Autodesk Inventor part; units mm, degrees
ref_plane "Work Plane1" through (0, 0, 0) normal (0, 0, 1) x (1, 0, 0)
ref_plane "Work Plane2" through (0, 0, 122.75) normal (0, 0, 1) x (1, 0, 0)
ref_plane "YZ Plane" through (0, 0, 0) normal (1, 0, 0) x (0, 1, 0)
ref_plane "Work Plane1" through (0, 0, 0) normal (0, 0, 1) x (1, 0, 0)
sketch "Sketch1" plane through (0, 0, 0) normal (0, 0, 1) x (1, 0, 0)
  line L0 (10, 0) -> (-1.5, 0)
  line L1 (10, 45.2667) -> (10, 0)
  arc A0 (13.0769, 49.8821) -> (10, 45.2667) centre (15, 45.2667) ccw
  line L2 (54.8615, 67.2923) -> (13.0769, 49.8821)
  line L3 (50.4385, 77.9077) -> (54.8615, 67.2923)
  line L4 (50.4385, 77.9077) -> (29.2692, 69.0872)
  arc A1 (29.2692, 69.0872) -> (-1.5, 22.9333) centre (48.5, 22.9333) ccw
  line L5 (-1.5, 0) -> (-1.5, 22.9333)
  line L6 (15, 45.2667) -> (6.8975, 50.6683)
  line L7 (10, 48.6) -> (19.7692, 25.1538)
  line L8 (35.4, 31.6667) -> (10, 21.0833)
  line L9 (19.1124, 26.7302) -> (10, 22.9333)
  line L10 (-1.5, 22.9333) -> (10, 22.9333)
  line L11 (-1.5, 22.9333) -> (0, 22.9333)
  line L12 (0, 22.9333) -> (0, -23.4445)
  line L13 (0, -23.4445) -> (-1.5, -23.4445)
  line L14 (-1.5, -23.4445) -> (-1.5, 22.9333)
  line L15 (0, 0.0333) -> (4, 0.0333)
  line L16 (4, 0.0333) -> (10, 6.0333)
  point P0 (0, 0)
  point P1 (10.4897, 47.4247)
  point P2 (10.8397, 48.0402)
  point P3 (10, 48.6)
  point P4 (0, 22.9333)
  dimension "d3" = 1.5
  dimension "d4" = 4
  dimension "d5" = 45
  dimension "d6" = 22.9
extrude "Extrusion1" add sketch "Sketch1" along normal blind 245.5 contours L16 L15 L12 L10 L1 | A1 L6 L7 A0 L1 L10 | L1 A0 L7 L9 | L6 A0 L7
sketch "Sketch2" plane through (6.8975, 50.6683, 245.5) normal (0.5547, 0.8321, 0) x (0.8321, -0.5547, 0)
  line L0 (4.738, 245.5) -> (0, 245.5)
  line L1 (0, 245.5) -> (0, 0)
  line L2 (4.738, 0) -> (0, 0)
  line L3 (4.738, 245.5) -> (4.738, 0)
  circle A0 centre (2.5, 230.5) radius 1.25
  circle A1 centre (2.5, 180.5) radius 1.25
  circle A2 centre (2.5, 130.5) radius 1.25
  circle A3 centre (2.5, 80.5) radius 1.25
  circle A4 centre (2.5, 30.5) radius 1.25
  point P0 (22.3667, 245.5)
  dimension "d7" = 2.5
  dimension "d8" = 2.5
  dimension "d9" = 15
  dimension "d12" = 50
extrude "Extrusion2" cut sketch "Sketch2" against normal blind 3 contours A0 | A1 | A2 | A3 | A4
sketch "Sketch3" plane through (0, 0, 0) normal (0, 0, -1) x (-1, 0, 0)
  line L0 (-10, 6.0333) -> (-10, 22.9333)
  line L1 (-4, 0.0333) -> (-10, 6.0333)
  line L2 (0, 0.0333) -> (-4, 0.0333)
  line L3 (0, 22.9333) -> (0, 0.0333)
  line L4 (1.5, 22.9333) -> (0, 22.9333)
  arc A0 (1.5, 22.9333) -> (-6.8975, 50.6683) centre (-48.5, 22.9333) ccw
  line L5 (-10.8397, 48.0402) -> (-6.8975, 50.6683)
  arc A1 (-10.4897, 47.4247) -> (-10.8397, 48.0402) centre (-15, 45.2667) ccw
  line L6 (-19.1124, 26.7302) -> (-10.4897, 47.4247)
  line L7 (-10, 22.9333) -> (-19.1124, 26.7302)
  line L8 (-12.4384, 34.9479) -> (-14.7461, 29.4095)
  line L9 (-14.7461, 29.4095) -> (-11.9768, 28.2556)
  line L10 (-11.9768, 28.2556) -> (-9.6691, 33.7941)
  line L11 (-9.6691, 33.7941) -> (-12.4384, 34.9479)
  point P0 (0, 0)
  dimension "d19" = 12.7
  dimension "d20" = 6
  dimension "d21" = 3
  dimension "d22" = 3
extrude "Extrusion3" cut sketch "Sketch3" against normal blind 30 contours L11 L10 L9 L8
sketch "Sketch4" plane through (10.4897, 47.4247, 245.5) normal (0.9231, 0.3846, 0) x (0, 0, -1)
  line L0 (245.5, -22.4191) -> (245.5, 0)
  line L1 (245.5, 0) -> (0, 0)
  line L2 (0, -22.4191) -> (0, 0)
  line L3 (245.5, -22.4191) -> (0, -22.4191)
  line L4 (245.5, -18.2665) -> (245.5, -12.2665) construction
  line L5 (245.5, -18.2665) -> (215.5, -18.2665)
  line L6 (215.5, -18.2665) -> (215.5, -12.2665)
  line L7 (245.5, -12.2665) -> (215.5, -12.2665)
  circle A0 centre (219.1, -15.2665) radius 1.65
  line L8 (220.7743, -18.1665) -> (217.4257, -18.1665)
  line L9 (217.4257, -18.1665) -> (215.7514, -15.2665)
  line L10 (215.7514, -15.2665) -> (217.4257, -12.3665)
  line L11 (217.4257, -12.3665) -> (220.7743, -12.3665)
  line L12 (220.7743, -12.3665) -> (222.4486, -15.2665)
  line L13 (222.4486, -15.2665) -> (220.7743, -18.1665)
  point P0 (245.5, -39.7422)
  point P1 (215.5, -15.2665)
  dimension "d25" = 3.3
  dimension "d26" = 3.6
  dimension "d27" = 5.8
extrude "Extrusion4" cut sketch "Sketch4" against normal blind 7 contours A0
ref_plane "Work Plane2" through (0, 0, 122.75) normal (0, 0, 1) x (1, 0, 0)
mirror "Mirror1" about plane through (0, 0, 122.75) normal (0, 0, 1) of "Extrusion4", "Extrusion3"
chamfer "Chamfer1" distance 3 angle 45 1 edges at (19.1124, 26.7302, 122.75)
properties part number "ESQUINA_REDONDEADA_R50_P2"
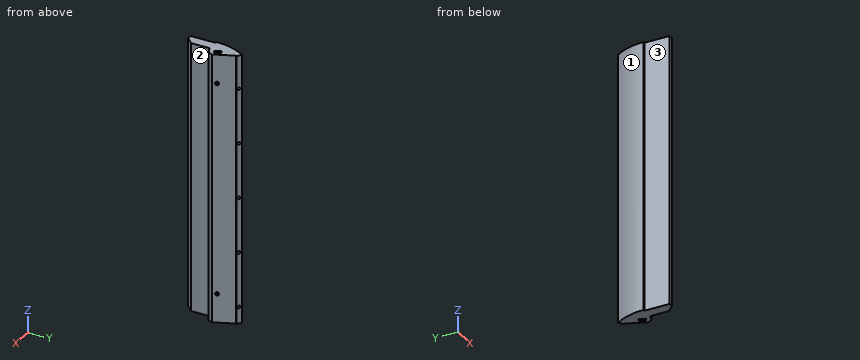
Geometry check sheet. Reference: the model listing, model coordinates, mm. Face numbers are marked on the shaded views. A direction names the side the tool comes from. Give positions to 0.01 mm unless a question says otherwise; leave off trailing zeros. Loops run counter-clockwise (first coordinate to the right, second up) from the corner with the lowest first, then second, coordinate; pieces in that order, holes last. Notation, with made-up numbers: (-28, 88.5) - (5, 88.5) arc R36 ccw to (5, 127.5) - close; hole circle Ø9 at (-16, -40). An arc over 180 degrees is marked (long way). Use CSV: the item, a comma, the result in double quotes. Start each with the question number.
Q1. Access from +Z, -Z, +X, -X, +Y, -Y to the whole of each face (thin tool, end or side, straight path). Record for the marked faces 1, 2 and 3.
Q2. Go/stop test with flat-tipped pins: pin 1 Ø5 at (x, z) = (15, 169.5) entering from +Y; pin 2 Ø1 at (y, z) = (35.5, 178.5) entering from -X; pin 3 Ø5 at (y, z) = (41, 144.5) entering from -X. Record where each tip stops, or that it passes through.
Q3. Scan lines: probe 1 along X at (y, z) = (14.5, 147); probe 2 along X at (y, z) = (39.5, 67); probe 3 along Y at (x, z) = (7, 50.5). Record each from-to range of solid material in increasing order. Write a range as from..to.
Q4. Section check C-C, the plane y = 41. Record the cut outline in (x, z).
Q5. Section check B-B, the plane y = 10. Record the cut outline in (x, z), and give its area (4 significant figures).
Q6. Section check A-A, the plane z = 92. Record the cut outline in (x, y), and give its area (3 significant figures).
Findings below:
1,face 1,"+Z, -Z, -X, +Y"
1,face 2,"+Z, -Z, +X, -Y"
1,face 3,"+Z, -Z, -X, -Y"
2,pin 1,"stops at y = 42.6"
2,pin 2,"stops at x = -0.02"
2,pin 3,"stops at x = 0.98"
3,probe 1,"x = 0..10"
3,probe 2,"x = 1.32..13.79"
3,probe 3,"y = 3.03..50.6"
4,outline,"(1.88, 0) - (13.17, 0) - (13.17, 245.5) - (1.88, 245.5) - close"
5,outline,"(0, 0) - (10, 0) - (10, 245.5) - (0, 245.5) - close"
5,area,"2,455 mm^2"
6,outline,"(-1.5, 22.93) - (0, 22.93) - (0, 0.03) - (4, 0.03) - (10, 6.03) - (10, 22.93) - (16.34, 25.58) - (17.96, 29.5) - (10.49, 47.42) arc R5 cw to (10.84, 48.04) - (6.9, 50.67) arc R50 ccw to start"
6,area,"565 mm^2"
